Read the model definition and answer for the solid it produces. Units are mm, in the model's axes. Give positions to 0.01 mm unless a question says otherwise; leave off trailing zeros. Loops run counter-clockwise (first coordinate to the right, second up) from the corner with the lowest first, then second, coordinate; pieces in that order, holes last.
(1) Each of these flat-tipped pins is pushed along its axis until it touches: P1, Ø2, axis at y = -1.5, z = 130.5, coming from the +X side; P2, Ø1.5, axis at x = -0.5, y = -2, coming from the +Z side; P3, Ø2, axis at x = 2.5, y = -0.5, coming from the -Z side. Where does it stop, or does it pass through?
(2) Find section A-A, the plane z = 14. Write down the section's boundary in (x, y), then the cut area to 3 significant figures.
(3) Straight lines are drawn through the part: probe 1 along Z at (x, y) = (1.75, 0.6); probe 2 along X at (y, z) = (-1.8, 25); probe 3 along X at (y, z) = (0.1, 51). For each, find the intervals that lie inside material, in ascending order.
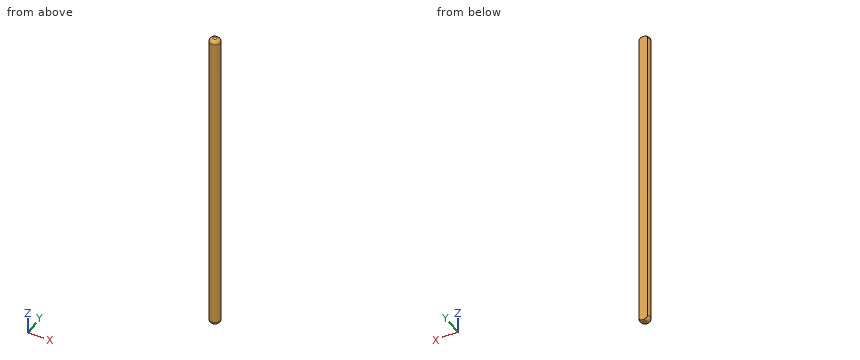
```python
from build123d import *

# Parameters (mm, degrees)
ESQUISSE1_R             = 3
BOSS_EXTRU_1_DEPTH      = 180
CONG_1_R                = 2
ESQUISSE2_W             = 6
ESQUISSE2_H             = 1.2
ENL_V_MAT_EXTRU_1_DEPTH = 181.049993057


with BuildPart() as part:
    # Esquisse1 → Boss.-Extru.1 (new body)
    with BuildSketch(Plane.XY):
        with Locations(Location((0, 0, 0), (0, 0, 180))):
            Circle(ESQUISSE1_R)
    extrude(amount=BOSS_EXTRU_1_DEPTH)

    # Congé1
    cong_1_edges = [part.edges().sort_by_distance(p)[0] for p in [
        (3, 0, 0),
        (3, 0, 180),
    ]]
    fillet(cong_1_edges, radius=CONG_1_R)

    # Esquisse2 → Enlèv. mat.-Extru.1 (cut, through all)
    with BuildSketch(Plane.XY.offset(180)):
        with Locations((0, 2.4)):
            Rectangle(ESQUISSE2_W, ESQUISSE2_H)
    extrude(amount=-ENL_V_MAT_EXTRU_1_DEPTH, mode=Mode.SUBTRACT)


solid = part.part
```
Entries:
1. P1: stops at x = 2.96
1. P2: stops at z = 179.98
1. P3: stops at z = 0.08
2. outline: (-2.4, 1.8) arc R3 ccw (long way) to (2.4, 1.8) - close
2. area: 24.2 mm2
3. probe 1: z = 0.19 to 179.81
3. probe 2: x = -2.4 to 2.4
3. probe 3: x = -3 to 3
